from build123d import *

# Parameters (mm, degrees)
ESQUISSE1_W             = 176.318824712
ESQUISSE1_H             = 111.873178338
BOSS_EXTRU_1_DEPTH      = 10
ESQUISSE2_W             = 111.873178338
ESQUISSE2_H             = 10
BOSS_EXTRU_3_DEPTH      = 10
ESQUISSE3_R             = 3.5
ENL_V_MAT_EXTRU_1_DEPTH = 10
ESQUISSE4_R             = 3.5
ENL_V_MAT_EXTRU_2_DEPTH = 10
ESQUISSE5_R             = 3.5
ENL_V_MAT_EXTRU_4_DEPTH = 10


with BuildPart() as part:
    # Esquisse1 → Boss.-Extru.1 (new body)
    with BuildSketch(Plane(origin=(0, 0, 0), x_dir=(0, 1, 0), z_dir=(0, 0, 1))):
        Rectangle(ESQUISSE1_W, ESQUISSE1_H)
    extrude(amount=BOSS_EXTRU_1_DEPTH)

    # Esquisse2 → Boss.-Extru.3 (add)
    with BuildSketch(Plane(origin=(0, 88.159412356, 0), x_dir=(-1, 0, 0), z_dir=(0, 1, 0))):
        with Locations((0, -5)):
            Rectangle(ESQUISSE2_W, ESQUISSE2_H)
    extrude(amount=-BOSS_EXTRU_3_DEPTH)

    # Esquisse3 → Enlèv. mat.-Extru.1 (cut)
    with BuildSketch(Plane.XZ.offset(-78.159412356)):
        with Locations(Location((11.791315902, -4.654466803, 0), (0, 0, 270))):
            Circle(ESQUISSE3_R)
        with Locations(Location((1.791315902, -4.654466803, 0), (0, 0, 270))):
            Circle(ESQUISSE3_R)
        with Locations(Location((-8.208684098, -4.654466803, 0), (0, 0, 270))):
            Circle(ESQUISSE3_R)
    extrude(amount=-ENL_V_MAT_EXTRU_1_DEPTH, mode=Mode.SUBTRACT)

    # Esquisse4 → Enlèv. mat.-Extru.2 (cut)
    with BuildSketch(Plane(origin=(0, 88.159412356, 0), x_dir=(-1, 0, 0), z_dir=(0, 1, 0))):
        with Locations(Location((-31.791315902, -4.654466803, 0), (0, 0, 90))):
            Circle(ESQUISSE4_R)
        with Locations(Location((28.208684098, -4.654466803, 0), (0, 0, 90))):
            Circle(ESQUISSE4_R)
    extrude(amount=-ENL_V_MAT_EXTRU_2_DEPTH, mode=Mode.SUBTRACT)

    # Esquisse5 → Enlèv. mat.-Extru.4 (cut)
    with BuildSketch(Plane(origin=(0, 88.159412356, 0), x_dir=(1, 0, 0), z_dir=(0, 1, 0))):
        with Locations(Location((-48.208684098, 4.654466803, 0), (0, 0, 270))):
            Circle(ESQUISSE5_R)
        with Locations(Location((51.791315902, 4.654466803, 0), (0, 0, 270))):
            Circle(ESQUISSE5_R)
    extrude(amount=-ENL_V_MAT_EXTRU_4_DEPTH, mode=Mode.SUBTRACT)


solid = part.part
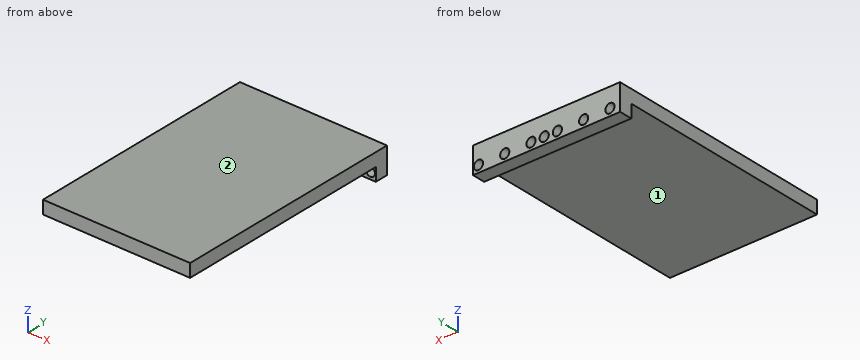
Design review of the part built by this model. Coordinates are the model's own, in mm. Face numbers are marked on the shaded views. A direction names the side the tool comes from. Give positions to 0.01 mm unless a question says otherwise; leave off trailing zeros. Loops run counter-clockwise (first coordinate to the right, second up) from the corner with the lowest first, then second, coordinate; pieces in that order, holes last. Notation, with made-up numbers: M -40,-11.75 L -17,-11.75 A17 ccw -17,11.25 Z; hole C 61,-27.5 d4. An arc over 180 degrees is marked long. Answer as a JSON object with one key per item and string values.
Item 1: We need section C-C (y = 4.5). State the section outline as (x, z) points, and give its area (3 significant figures).
Output values:
{"outline": "M -55.94,0 L 55.94,0 L 55.94,10 L -55.94,10 Z", "area": "1,120 mm2"}
Item 2: Machinability: for the marked faces 1 and 2, which of the approach directions +Z, -Z, +X, -X, +Y, -Y give a long, thin tool a straight path to every point of the face, cutting with its end or side? Answer none if there is none.
Output values:
{"face 1": "-Z, +X, -X, -Y", "face 2": "+Z, +X, -X, +Y, -Y"}
Item 3: We need section B-B (x = 25). State the section outline as (y, z) points.
Output values:
{"outline": "M -88.16,0 L 78.16,0 L 78.16,-10 L 88.16,-10 L 88.16,10 L -88.16,10 Z"}
Item 4: We need section A-A (z = -5). Count the separate pieces of the cut face and the enclosed holes in it, and give its area (3 significant figures).
Output values:
{"separate pieces": "8", "enclosed holes": "0", "area": "631 mm2"}
Item 5: For P1, Ø6.5, axis at x = 51.79, z = -4.65, coming from the +Y side; P2, Ø5, axis at x = -15.5, z = -6.5, coming from the -Y side; P3, Ø5, axis at x = 22.5, y = -40, coming from the -Z side, all flat-tipped, find the tip position at first contact; note any pin that passes through.
Output values:
{"P1": "passes through", "P2": "stops at y = 78.16", "P3": "stops at z = 0"}
Item 6: Wall thickness on line 1 along Z through (x, y) = (30, 27.5); line 2 along Y through (x, z) = (5, -8); line 3 along Z through (x, y) = (-49.5, 81.5): over which ranges is each line inside the solid? List them lowest first.
Output values:
{"line 1": "z = 0 to 10", "line 2": "y = 78.16 to 88.16", "line 3": "z = -10 to -7.91, -1.4 to 10"}
